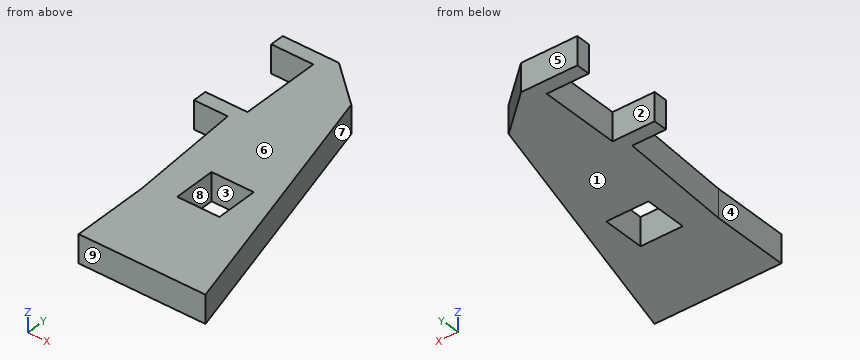
from build123d import *

# Parameters (mm, degrees)
BOSS_EXTRUDE1_DEPTH = 25.4
SKETCH2_W           = 38.1
SKETCH2_H           = 38.1
CUT_EXTRUDE1_DEPTH  = 303.885239179


with BuildPart() as part:
    # Sketch1 → Boss-Extrude1 (new body)
    with BuildSketch(Plane.XY):
        Polygon((0, 0), (0, 12.7), (50.8, 12.7), (88.9, -20.510228633), (152.4, -260.515926793), (38.018659419, -260.515926793), (38.018659419, -190.696503564), (30.48, -85.763926793), (0, -85.763926793), (0, -73.152260366), (38.018659419, -73.152260366), (38.018659419, 0), align=None)
    extrude(amount=BOSS_EXTRUDE1_DEPTH)

    # Sketch2 → Cut-Extrude1 (cut, through all)
    with BuildSketch(Plane(origin=(0, 0, 0), x_dir=(-1, 0, 0), z_dir=(0, 0, -1))):
        with Locations((-82.574564704, -163.487926793)):
            Rectangle(SKETCH2_W, SKETCH2_H)
    extrude(amount=-CUT_EXTRUDE1_DEPTH, mode=Mode.SUBTRACT)


solid = part.part
Design review of the part built by this model. Coordinates are the model's own, in mm. Face numbers are marked on the shaded views. A direction names the side the tool comes from. Give positions to 0.01 mm unless a question says otherwise; leave off trailing zeros. Order: outer loops, then holes, each group sorted by start corner. A loop starts at its lowest first (then second) coordinate and runs counter-clockwise, first axis right, second up.
1. Add section D-D, the plane y = -221.5. State the section outline as (x, z) points.
Solution:
outline: (38.02, 0) - (142.08, 0) - (142.08, 25.4) - (38.02, 25.4) - close
2. Add section A-A, the plane z = 4.25. State the section outline as (x, y) points.
Solution:
outline: (0, -85.76) - (30.48, -85.76) - (38.02, -190.7) - (38.02, -260.52) - (152.4, -260.52) - (88.9, -20.51) - (50.8, 12.7) - (0, 12.7) - (0, 0) - (38.02, 0) - (38.02, -73.15) - (0, -73.15) - close; hole (63.52, -182.54) - (101.62, -182.54) - (101.62, -144.44) - (63.52, -144.44) - close
3. For pin 1 Ø12.5 at (x, z) = (19, 8.5) entering from -Y; pin 2 Ø6 at (y, z) = (-178.5, 10.5) entering from -X; pin 3 Ø7.5 at (y, z) = (-171.5, 8.5) entering from +X, all flat-tipped, find the tip position at first contact; note any pin that passes through.
Solution:
pin 1: stops at y = -85.76
pin 2: stops at x = 36.93
pin 3: stops at x = 129.84
4. Add section C-C, the plane y = -169. State the section outline as (x, z) points.
Solution:
outline: (36.46, 0) - (63.52, 0) - (63.52, 25.4) - (36.46, 25.4) - close; (101.62, 0) - (128.19, 0) - (128.19, 25.4) - (101.62, 25.4) - close
5. Tool access review of the marked faces 1, 2, 3, 4 and 5: name each direction out of +Z, -Z, +X, -X, +Y, -Y from which nothing blocks a thin tool from reaching the whole face with its end or side.
Solution:
face 1: -Z, +X, -X, +Y, -Y
face 2: +Z, -Z, -X
face 3: +Z, -Z
face 4: +Z, -Z, -X, -Y
face 5: +Z, -Z, +X, -X, +Y
6. Mouldability with a two-part tool opening along Y and no side actions: class the marked faces 6, 7, 8 and 9 as +Y half, -Y half, draft (parallel to the pull), parting line (faces both ways), or undercut.
Solution:
face 6: draft
face 7: +Y half
face 8: undercut
face 9: -Y half
7. Add section B-B, the plane x = 15. State the section outline as (y, z) points.
Solution:
outline: (-85.76, 0) - (-73.15, 0) - (-73.15, 25.4) - (-85.76, 25.4) - close; (0, 0) - (12.7, 0) - (12.7, 25.4) - (0, 25.4) - close
8. To check wall thickness, follow L1, parallel to Y at x = 71, z = 23.5; L2, parallel to Y at x = 84.5, z = 17.25; L3, parallel to X at y = -24.5, z = 10.75. State the ranges of each line that lie inside material, in increasing order.
Solution:
L1: y = -260.52 to -182.54, -144.44 to -4.91
L2: y = -260.52 to -182.54, -144.44 to -16.67
L3: x = 38.02 to 89.96
